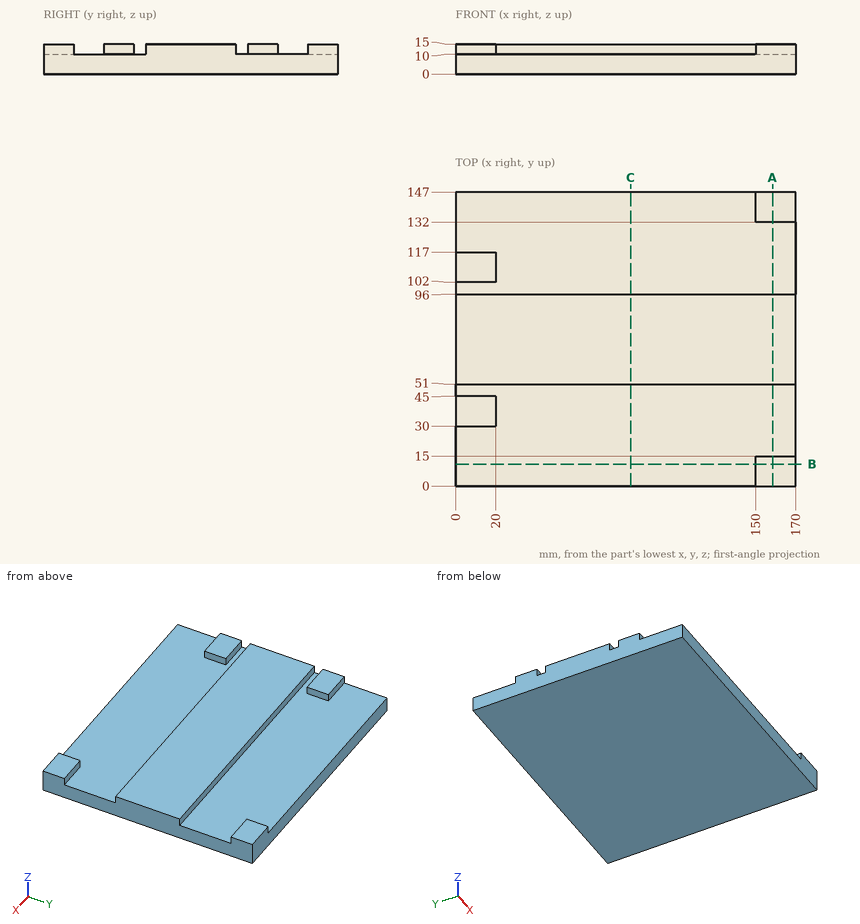
Study the drawing (mm; zero at the part's minimum x, y, z) and answer. Give positions to 0.01 mm unless a question says otherwise; leave off trailing zeros. Write each loop counter-clockwise with the first axis right and the second up, starting at its lowest first coordinate (ties: lowest second). Pieces come first, ordered by that corner, then holes. Notation, with made-up numbers: (0, 38) - (50, 38) arc R28 ccw to (50, 61) - close; hole circle Ø6 at (28, 39.5). An arc over 180 degrees is marked (long way). Write item = value, one per line. Start each with the question number.
Item 1: Find section B-B (y = 11). Give the vertices of the cut face in (x, z), then the cut area to 3 significant figures.
Item 2: Find the intervals of material crossed by probe 1 along Y at (x, z) = (9, 14); probe 2 along Y at (x, z) = (39, 10.5); probe 3 along Z at (x, y) = (75, 28.5), in increasing order. Write a range as [from, to].
Item 3: Each of these flat-tipped pins is pushed along its axis until it touches: P1, Ø1.5, axis at y = 109.5, z = 11.5, coming from the +X side; P2, Ø4, axis at x = 79.5, z = 13.5, coming from the -Y side; P3, Ø2.5, axis at x = 7, z = 13, coming from the -Y side. Where does it stop, or does it pass through?
Item 4: Find section A-A (x = 158.5). Give the vertices of the cut face in (y, z).
Item 5: Find section C-C (x = 87.5). Give the vertices of the cut face in (y, z), then the cut area to 4 significant figures.
Response:
q1.outline = (0, 0) - (170, 0) - (170, 15) - (150, 15) - (150, 10) - (0, 10) - close
q1.area = 1,800 mm²
q2.probe_1 = [30, 45], [51, 96], [102, 117]
q2.probe_2 = [51, 96]
q2.probe_3 = [0, 10]
q3.P1 = 20
q3.P2 = 51
q3.P3 = 30
q4.outline = (0, 0) - (147, 0) - (147, 15) - (132, 15) - (132, 10) - (96, 10) - (96, 15) - (51, 15) - (51, 10) - (15, 10) - (15, 15) - (0, 15) - close
q5.outline = (0, 0) - (147, 0) - (147, 10) - (96, 10) - (96, 15) - (51, 15) - (51, 10) - (0, 10) - close
q5.area = 1,695 mm²
